Here's how the part is built. I have some questions about the finished solid (model axes, mm). Round coordinates to 2 decimals unless told otherwise and drop trailing zeros. Loops run counter-clockwise (first coordinate to the right, second up) from the corner with the lowest first, then second, coordinate; pieces in that order, holes last. Notation, with made-up numbers: M 80.25,71.25 L 103.25,71.25 A32 ccw 103.25,101.25 Z; hole C -32.5,34.25 d2. An arc over 180 degrees is marked long. Answer as a JSON object with one key per item and string values.
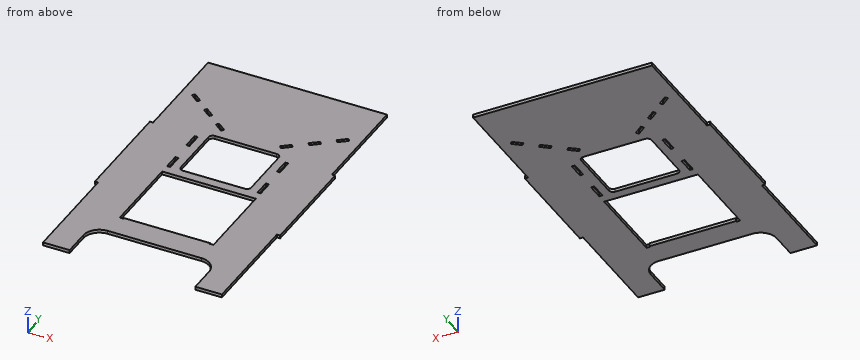
Autodesk Inventor part; units mm, degrees
ref_plane "YZ Plane" through (0, 0, 0) normal (1, 0, 0) x (0, 1, 0)
ref_plane "XZ Plane" through (0, 0, 0) normal (0, 1, 0) x (-1, 0, 0)
ref_plane "XY Plane" through (0, 0, 0) normal (0, 0, 1) x (1, 0, 0)
sketch "Sketch1" plane through (0, 0, 0) normal (0, 0, 1) x (1, 0, 0)
  line L0 (-76.9983, 8.3713) -> (-75.1513, 10.7353)
  line L1 (-75.1513, 10.7353) -> (-67.2712, 4.5787)
  line L2 (-67.2712, 4.5787) -> (-69.1182, 2.2147)
  line L3 (-69.1182, 2.2147) -> (-76.9983, 8.3713)
  line L4 (-86.1834, 19.3546) -> (-88.0304, 16.9906)
  line L5 (-88.0304, 16.9906) -> (-95.9105, 23.1472)
  line L6 (-95.9105, 23.1472) -> (-94.0636, 25.5112)
  line L7 (-94.0636, 25.5112) -> (-86.1834, 19.3546)
  line L8 (-106.9427, 31.7664) -> (-114.8228, 37.9231)
  line L9 (-114.8228, 37.9231) -> (-112.9758, 40.2871)
  line L10 (-112.9758, 40.2871) -> (-105.0957, 34.1305)
  line L11 (-105.0957, 34.1305) -> (-106.9427, 31.7664)
  line L12 (-6.8487, 10.7353) -> (-5.0017, 8.3713)
  line L13 (-5.0017, 8.3713) -> (-12.8818, 2.2147)
  line L14 (-12.8818, 2.2147) -> (-14.7288, 4.5787)
  line L15 (-14.7288, 4.5787) -> (-6.8487, 10.7353)
  line L16 (6.0304, 16.9906) -> (4.1834, 19.3546)
  line L17 (4.1834, 19.3546) -> (12.0636, 25.5112)
  line L18 (12.0636, 25.5112) -> (13.9105, 23.1472)
  line L19 (13.9105, 23.1472) -> (6.0304, 16.9906)
  line L20 (32.8228, 37.9231) -> (24.9427, 31.7664)
  line L21 (24.9427, 31.7664) -> (23.0957, 34.1305)
  line L22 (23.0957, 34.1305) -> (30.9758, 40.2871)
  line L23 (30.9758, 40.2871) -> (32.8228, 37.9231)
  line L24 (-82, 0) -> (-82, -73.9786) construction
  line L25 (-82, -73.9786) -> (-82, -147.5817) construction
  line L26 (-82, -147.5817) -> (-85, -147.5817)
  line L27 (-85, -147.5817) -> (-85, -73.9786)
  line L28 (-85, -73.9786) -> (-85, 0) construction
  line L29 (-85, 0) -> (-82, 0) construction
  line L30 (-85, -73.9786) -> (-82, -73.9786)
  line L31 (3, 0) -> (3, -73.9786) construction
  line L32 (3, -73.9786) -> (3, -147.5817)
  line L33 (3, -147.5817) -> (0, -147.5817)
  line L34 (0, -147.5817) -> (0, -73.9786) construction
  line L35 (0, -73.9786) -> (0, 0) construction
  line L36 (0, 0) -> (3, 0) construction
  line L37 (0, -73.9786) -> (3, -73.9786)
  line L38 (-82, -143.7746) -> (0, -143.7746) construction
  line L39 (0, -143.7746) -> (0, -147.5817)
  line L40 (0, -147.5817) -> (-82, -147.5817)
  line L41 (-82, -147.5817) -> (-82, -143.7746)
  line L42 (-82, -73.9786) -> (0, -73.9786)
  line L43 (-85, -65) -> (-85, -50)
  line L44 (-85, -50) -> (-82, -50)
  line L45 (-82, -50) -> (-82, -65)
  line L46 (-82, -65) -> (-85, -65)
  line L47 (3, -50) -> (3, -65)
  line L48 (3, -65) -> (0, -65)
  line L49 (0, -65) -> (0, -50)
  line L50 (0, -50) -> (3, -50)
  line L51 (-82, -30) -> (-85, -30)
  line L52 (-85, -30) -> (-85, -15)
  line L53 (-85, -15) -> (-82, -15)
  line L54 (-82, -15) -> (-82, -30)
  line L55 (3, -30) -> (0, -30)
  line L56 (0, -30) -> (0, -15)
  line L57 (0, -15) -> (3, -15)
  line L58 (3, -15) -> (3, -30)
  line L59 (43, 87) -> (-125, 87)
  line L60 (-128, -13) -> (-128, -113)
  line L61 (18, -213) -> (43, -213)
  line L62 (46, -113) -> (46, -13)
  line L63 (-125, -113) -> (-125, -213)
  line L64 (43, -213) -> (43, -113)
  line L65 (43, -113) -> (46, -113)
  line L66 (46, -13) -> (43, -13)
  line L67 (43, -13) -> (43, 87)
  line L68 (-125, 87) -> (-125, -13)
  line L69 (-125, -13) -> (-128, -13)
  line L70 (-128, -113) -> (-125, -113)
  line L71 (-100, -213) -> (-100, -188)
  arc A0 (-85, -173) -> (-100, -188) centre (-85, -188) ccw
  line L72 (-85, -173) -> (3, -173)
  arc A1 (18, -188) -> (3, -173) centre (3, -188) ccw
  line L73 (18, -188) -> (18, -213)
  line L74 (-125, -213) -> (-100, -213)
extrude "Extrusion1" add sketch "Sketch1" along normal blind 3
sketch "Sketch2" plane through (0, 0, 3) normal (0, 0, 1) x (1, 0, 0)
  line L0 (-82, -76.3225) -> (-82, -149.9255)
  line L1 (-82, -149.9255) -> (-85, -149.9255)
  line L2 (-85, -149.9255) -> (-85, -76.3225)
  line L3 (-85, -76.3225) -> (-82, -76.3225)
  line L4 (-82, -146.1185) -> (0, -146.1185)
  line L5 (0, -146.1185) -> (0, -149.9255)
  line L6 (0, -149.9255) -> (-82, -149.9255)
  line L7 (-82, -149.9255) -> (-82, -146.1185)
  line L8 (3, -76.3225) -> (3, -149.9255)
  line L9 (3, -149.9255) -> (0, -149.9255)
  line L10 (0, -149.9255) -> (0, -76.3225)
  line L11 (0, -76.3225) -> (3, -76.3225)
  point P0 (0, 0)
extrude "Extrusion2" cut sketch "Sketch2" against normal blind 10
sketch "Sketch4" plane through (0, 0, 3) normal (0, 0, 1) x (1, 0, 0)
  line L0 (-85, -149.9255) -> (3, -149.9255)
  line L1 (-85, -149.9255) -> (3, -149.9255)
  line L2 (3, -149.9255) -> (3, -150.9255)
  line L3 (3, -150.9255) -> (-85, -150.9255)
  line L4 (-85, -150.9255) -> (-85, -149.9255)
  line L5 (3, -73.9786) -> (3, -149.9255)
  line L6 (3, -149.9255) -> (-85, -149.9255)
  line L7 (-0.5, -149.9255) -> (-0.5, -150.9255)
  line L8 (-81.5, -149.9255) -> (-81.5, -150.9255)
  point P0 (0, 0)
  point P1 (3, -149.9255)
  dimension "d6" = 1
  dimension "d22" = 3.5
  dimension "d23" = 3.5
extrude "Extrusion4" cut sketch "Sketch4" against normal blind 10 contours L0 L8 L3 L4 | L0 L2 L3 L7
sketch "Sketch6" plane through (0, 0, 3) normal (0, 0, 1) x (1, 0, 0)
  line L0 (-100, -213) -> (18, -213)
  line L1 (18, -213) -> (18, -173)
  line L2 (18, -173) -> (-100, -173)
  line L3 (-100, -173) -> (-100, -213)
  line L4 (-125, -113) -> (-125, -213)
  line L5 (43, -213) -> (43, -113)
  line L6 (-125, -213) -> (43, -213)
  point P0 (0, 0)
  dimension "d9" = 25
  dimension "d10" = 25
  dimension "d11" = 40
extrude "Extrusion5" cut sketch "Sketch6" against normal blind 10
fillet "Fillet1" radius 15 2 edges at (-100, -173, 1.5) (18, -173, 1.5)
sketch "Sketch7" plane through (0, 0, 3) normal (0, 0, 1) x (1, 0, 0)
  line L0 (-74, -64.9786) -> (-8, -64.9786)
  line L1 (-8, -64.9786) -> (-8, -6.9786)
  line L2 (-8, -6.9786) -> (-74, -6.9786)
  line L3 (-74, -6.9786) -> (-74, -64.9786)
  line L4 (0, -65) -> (0, -50)
  line L5 (-82, -50) -> (-82, -65)
  line L6 (-85, -73.9786) -> (3, -73.9786)
  dimension "d15" = 8
  dimension "d16" = 8
  dimension "d17" = 9
  dimension "d18" = 58
extrude "Extrusion6" cut sketch "Sketch7" against normal blind 10
fillet "Fillet2" radius 4 4 edges at (-74, -6.9786, 1.5) (-8, -6.9786, 1.5) (-8, -64.9786, 1.5) (-74, -64.9786, 1.5)
properties part number "Pared_Frontal"
Item 1: If I drill on L1, parallel to Y at x = -15, z = 1.3; L2, parallel to X at y = -46, z = 2.2; L3, parallel to Y at x = -68, z = 1.7, over which ranges is the centre line in solid material (lowest first)? Write a range as from..to.
Solution:
{"L1": "y = -173..-149.93, -73.98..-64.98, -6.98..87", "L2": "x = -128..-74, -8..46", "L3": "y = -173..-149.93, -73.98..-64.98, -6.98..3.65, 5.15..87"}
Item 2: I want a section at C-C on y = -24. List the corners of the cut face in (x, z) for me, plus the area to 3 significant figures.
Solution:
{"outline": "M -128,0 L -85,0 L -85,3 L -128,3 Z; M -82,0 L -74,0 L -74,3 L -82,3 Z; M -8,0 L 0,0 L 0,3 L -8,3 Z; M 3,0 L 46,0 L 46,3 L 3,3 Z", "area": "306 mm2"}
Item 3: I want a section at D-D on z = 1.05. Count the separate pieces of the cut face and the enclosed holes in it, plus the area to 3 significant figures.
Solution:
{"separate pieces": "1", "enclosed holes": "12", "area": "35,500 mm2"}
Item 4: I want a section at A-A on y = -129. List the corners of the cut face in (x, z) for me, plus the area to 3 significant figures.
Solution:
{"outline": "M -125,0 L -85,0 L -85,3 L -125,3 Z; M 3,0 L 43,0 L 43,3 L 3,3 Z", "area": "240 mm2"}
Item 5: For P1, Ø0.9, axis at x = 44, z = 1.5, coming from the +Y side; P2, Ø1.5, axis at y = -155.5, z = 1.5, coming from the -X side; P3, Ø1.5, axis at y = -205.5, z = 1.5, coming from the +X side, each with a flat end and sliding along its axis, tell me the tip position at first contact or that it passes through.
Solution:
{"P1": "stops at y = -13", "P2": "stops at x = -125", "P3": "stops at x = 43"}
Item 6: I want a section at B-B on x = -35. List the corners of the cut face in (y, z) for me.
Solution:
{"outline": "M -173,0 L -149.93,0 L -149.93,3 L -173,3 Z; M -73.98,0 L -64.98,0 L -64.98,3 L -73.98,3 Z; M -6.98,0 L 87,0 L 87,3 L -6.98,3 Z"}
